For this review, use the dimensioned drawing (mm, ordinates from the lowest corner) and the shaded views. Round coordinates to 2 decimals unless told otherwise and drop trailing zeros. Write each question's results on one line, items separated by ' | '.
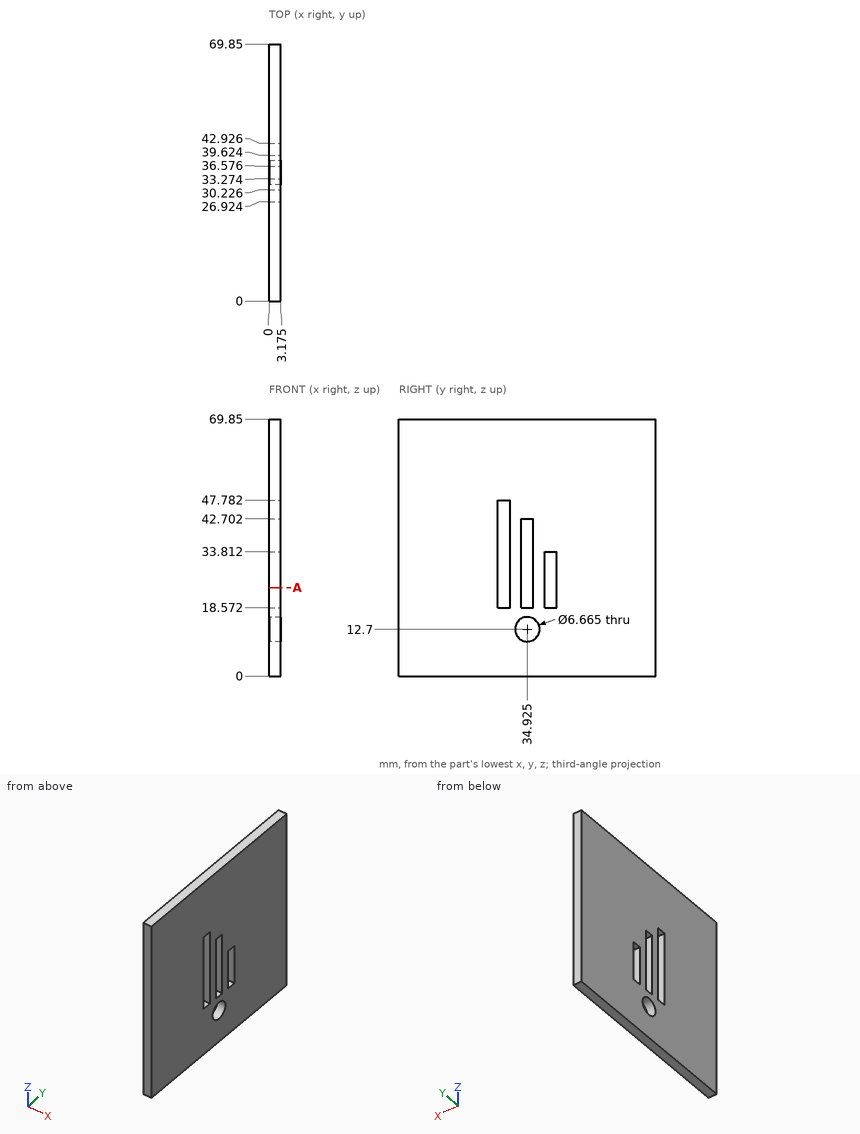
1. For pin 1 (1 mm diameter, centred on y = 35.5, z = 24.5, fed in from +X), flat-tipped, find the tip position at first contact; note if it passes through.
Values found:
pin 1: passes through
2. Consider section A-A (z = 24). Give the number of separate pieces and of enclosed holes in the cut face, plus the area to 3 significant figures.
Values found:
separate pieces: 4 | enclosed holes: 0 | area: 190 mm2
3. To check wall thickness, follow probe 1 along Y at (x, z) = (2.45, 26.5); probe 2 along Y at (x, z) = (1.6, 45); probe 3 along Z at (x, y) = (1.2, 41). State the ranges of each line that lie inside material, in increasing order.
Values found:
probe 1: y = 0 to 26.92, 30.23 to 33.27, 36.58 to 39.62, 42.93 to 69.85 | probe 2: y = 0 to 26.92, 30.23 to 69.85 | probe 3: z = 0 to 18.57, 33.81 to 69.85
